```python
from build123d import *

# Parameters (mm, degrees)
SKETCH1_R                       = 48.5
SKETCH1_R_2                     = 1.5
BOSS_EXTRUDE3_DEPTH             = 4
BOSS_EXTRUDE4_START             = 4
SKETCH3_R                       = 9
BOSS_EXTRUDE4_DEPTH             = 14
CUT_EXTRUDE2_START              = 6
SKETCH5_R                       = 1.3
CUT_EXTRUDE2_DEPTH              = 96.333743786
BOSS_EXTRUDE5_DEPTH             = 9
BOSS_EXTRUDE5_DIRECTION_2_REACH = 113.079
CUT_EXTRUDE3_DEPTH              = 107.628687584
CUT_EXTRUDE3_DEPTH_BACK         = 107.628687584
FILLET1_R                       = 10
FILLET2_R                       = 2
SKETCH11_R                      = 3.75
CUT_EXTRUDE4_DEPTH              = 2.6


with BuildPart() as part:
    # Sketch1 → Boss-Extrude3 (new body)
    with BuildSketch(Plane(origin=(0, 0, 0), x_dir=(1, 0, 0), z_dir=(0, 1, 0))):
        with Locations(Location((0, 0, 0), (0, 0, 270))):
            Circle(SKETCH1_R)
        with Locations(Location((0, 7.25, 0), (0, 0, 270))):
            Circle(SKETCH1_R_2, mode=Mode.SUBTRACT)
        with Locations(Location((0, -7.25, 0), (0, 0, 270))):
            Circle(SKETCH1_R_2, mode=Mode.SUBTRACT)
    extrude(amount=BOSS_EXTRUDE3_DEPTH)

    # Sketch3 → Boss-Extrude4 (add)
    with BuildSketch(Plane(origin=(0, 0, 0), x_dir=(0, 0, -1), z_dir=(1, 0, 0)).offset(BOSS_EXTRUDE4_START)):
        with BuildLine():
            Line((30.34, 4), (-30.34, 4))
            Line((-30.34, 4), (-30.34, 11.86))
            ThreePointArc((-30.34, 11.86), (-29.573286886, 19.169908139), (-27.306519614, 26.161644128))
            Line((-27.306519614, 26.161644128), (-13.792358873, 56.58534489))
            ThreePointArc((-13.792358873, 56.58534489), (31.303559207, 69.105517077), (34.935565542, 22.444986978))
            ThreePointArc((34.935565542, 22.444986978), (31.536621485, 17.510838233), (30.34, 11.64))
            Line((30.34, 11.64), (30.34, 4))
        make_face()
        with Locations((13.91, 44.28)):
            Circle(SKETCH3_R, mode=Mode.SUBTRACT)
    extrude(amount=BOSS_EXTRUDE4_DEPTH)

    # Sketch5 → Cut-Extrude2 (cut, through all)
    with BuildSketch(Plane(origin=(0, 0, 0), x_dir=(0, 0, -1), z_dir=(1, 0, 0)).offset(CUT_EXTRUDE2_START)):
        with Locations(Location((27.167164466, 50.465339059, 0), (0, 0, 180))):
            Circle(SKETCH5_R)
        with Locations(Location((20.096096654, 57.536406871, 0), (0, 0, 180))):
            Circle(SKETCH5_R)
        with Locations(Location((-6.773961031, 16.524213562, 0), (0, 0, 180))):
            Circle(SKETCH5_R)
        with Locations(Location((-13.845028843, 23.595281374, 0), (0, 0, 180))):
            Circle(SKETCH5_R)
        Polygon((-0.41, 15.11), (28.581378029, 44.101378029), (13.732135624, 58.950620434), (-15.259242405, 29.959242405), align=None)
    extrude(amount=CUT_EXTRUDE2_DEPTH, mode=Mode.SUBTRACT)

    # Sketch9 → Boss-Extrude5 (add)
    with BuildSketch(Plane(origin=(18, 0, 0), x_dir=(0, 0, -1), z_dir=(1, 0, 0))):
        with BuildLine():
            Line((30.34, 4), (30.34, 11.64))
            ThreePointArc((30.34, 11.64), (31.536621485, 17.510838233), (34.935565542, 22.444986978))
            ThreePointArc((34.935565542, 22.444986978), (31.303559207, 69.105517077), (-13.792358873, 56.58534489))
            ThreePointArc((-13.792358873, 56.58534489), (-24.20389685, 31.229863028), (-27.34, 4))
            Line((-27.34, 4), (-36.34, 4))
            Line((-36.34, 4), (-36.34, 11.86))
            ThreePointArc((-36.34, 11.86), (-35.442708439, 20.414854175), (-32.789889403, 28.597348492))
            Line((-32.789889403, 28.597348492), (-19.275728663, 59.021049255))
            ThreePointArc((-19.275728663, 59.021049255), (34.746418262, 74.019448449), (39.097339325, 18.122992187))
            ThreePointArc((39.097339325, 18.122992187), (37.057972891, 15.16250294), (36.34, 11.64))
            Line((36.34, 11.64), (36.34, 4))
            Line((36.34, 4), (30.34, 4))
        make_face()
    extrude(amount=BOSS_EXTRUDE5_DEPTH)

    # Boss-Extrude5 direction 2: up to this face of the body (flat: up to its plane)
    boss_extrude5_direction_2_end = Plane(part.part.faces().sort_by_distance((4, 35.761181815, -7.797700276))[0])
    # Sketch9 → Boss-Extrude5 direction 2 (add, up to the picked face)
    with BuildSketch(Plane(origin=(18, 0, 0), x_dir=(0, 0, -1), z_dir=(1, 0, 0)), mode=Mode.PRIVATE) as boss_extrude5_direction_2_sk1:
        with BuildLine():
            Line((30.34, 4), (30.34, 11.64))
            ThreePointArc((30.34, 11.64), (31.536621485, 17.510838233), (34.935565542, 22.444986978))
            ThreePointArc((34.935565542, 22.444986978), (31.303559207, 69.105517077), (-13.792358873, 56.58534489))
            ThreePointArc((-13.792358873, 56.58534489), (-24.20389685, 31.229863028), (-27.34, 4))
            Line((-27.34, 4), (-36.34, 4))
            Line((-36.34, 4), (-36.34, 11.86))
            ThreePointArc((-36.34, 11.86), (-35.442708439, 20.414854175), (-32.789889403, 28.597348492))
            Line((-32.789889403, 28.597348492), (-19.275728663, 59.021049255))
            ThreePointArc((-19.275728663, 59.021049255), (34.746418262, 74.019448449), (39.097339325, 18.122992187))
            ThreePointArc((39.097339325, 18.122992187), (37.057972891, 15.16250294), (36.34, 11.64))
            Line((36.34, 11.64), (36.34, 4))
            Line((36.34, 4), (30.34, 4))
        make_face()
    boss_extrude5_direction_2_tool1 = split(extrude(boss_extrude5_direction_2_sk1.sketch, amount=-BOSS_EXTRUDE5_DIRECTION_2_REACH, mode=Mode.PRIVATE), bisect_by=boss_extrude5_direction_2_end, keep=Keep.BOTH, mode=Mode.PRIVATE)
    add(boss_extrude5_direction_2_tool1.solids().sort_by(Axis((18, 43.339989, 24.976501), (-1, 0, 0)))[0])

    # Sketch10 → Cut-Extrude3 (cut, two sides: drawn at the far end of the back side and taken through both)
    with BuildSketch(Plane.XY.offset(-CUT_EXTRUDE3_DEPTH_BACK)):
        with BuildLine():
            Line((27, 80.59241), (21, 80.59241))
            ThreePointArc((21, 80.59241), (22.277450308, 42.190463148), (26.5, 4))
            Line((26.5, 4), (27, 4))
            Line((27, 4), (27, 80.59241))
        make_face()
    extrude(amount=CUT_EXTRUDE3_DEPTH + CUT_EXTRUDE3_DEPTH_BACK, mode=Mode.SUBTRACT)

    # Fillet1
    # the kernel refuses this fillet: 10 mm, written as the material it takes off along each edge
    with BuildSketch(Plane(origin=(4, 11.64, -36.34), x_dir=(0, 0, 1), z_dir=(0, -1, 0))) as fillet1_piece_1:
        with BuildLine():
            CenterArc((FILLET1_R, -FILLET1_R), FILLET1_R, 90, 90)
            Line((0, -FILLET1_R), (0, 0))
            Line((0, 0), (FILLET1_R, 0))
        make_face()
    extrude(amount=7.64, mode=Mode.SUBTRACT)
    with BuildSketch(Plane(origin=(4, 11.64, -45.34), x_dir=(0, 0.7203324652134895, 0.6936289638988969), z_dir=(0, 0.6936289638988969, -0.7203324652134895))) as fillet1_piece_2:
        with BuildLine():
            CenterArc((9 + FILLET1_R, FILLET1_R), FILLET1_R, 180, 90)
            Line((9, FILLET1_R), (9, 0))
            Line((9, 0), (9 + FILLET1_R, 0))
        make_face()
    revolve(axis=Axis((4, 11.64, -45.34), (1, 0, 0)), revolution_arc=46.081936205, mode=Mode.SUBTRACT)
    with BuildSketch(Plane(origin=(4, 44.28, -13.91), x_dir=(0, -0.7203324652134897, -0.6936289638988965), z_dir=(0, -0.6936289638988965, 0.7203324652134897))) as fillet1_piece_3:
        with BuildLine():
            CenterArc((36.31241 - FILLET1_R, FILLET1_R), FILLET1_R, 270, 90)
            Line((36.31241, FILLET1_R), (36.31241, 0))
            Line((36.31241, 0), (36.31241 - FILLET1_R, 0))
        make_face()
    revolve(axis=Axis((4, 44.28, -13.91), (1, 0, 0)), revolution_arc=202.131217863, mode=Mode.SUBTRACT)
    with BuildSketch(Plane(origin=(4, 28.597348492, 32.789889403), x_dir=(0, -0.40595072743967076, -0.913894964911834), z_dir=(0, 0.913894964911834, -0.4059507274396708))) as fillet1_piece_4:
        with BuildLine():
            CenterArc((FILLET1_R, -FILLET1_R), FILLET1_R, 90, 90)
            Line((0, -FILLET1_R), (0, 0))
            Line((0, 0), (FILLET1_R, 0))
        make_face()
    extrude(amount=33.290150324, mode=Mode.SUBTRACT)
    with BuildSketch(Plane(origin=(4, 11.86, -4.89), x_dir=(0, 0.4059507274396698, 0.9138949649118343), z_dir=(0, 0.9138949649118343, -0.4059507274396698))) as fillet1_piece_5:
        with BuildLine():
            CenterArc((41.23 - FILLET1_R, FILLET1_R), FILLET1_R, 270, 90)
            Line((41.23, FILLET1_R), (41.23, 0))
            Line((41.23, 0), (41.23 - FILLET1_R, 0))
        make_face()
    revolve(axis=Axis((4, 11.86, -4.89), (1, 0, 0)), revolution_arc=23.950718343, mode=Mode.SUBTRACT)
    with BuildSketch(Plane(origin=(4, 4, 36.34), x_dir=(0, 0, -1), z_dir=(0, 1, 0))) as fillet1_piece_6:
        with BuildLine():
            CenterArc((FILLET1_R, -FILLET1_R), FILLET1_R, 90, 90)
            Line((0, -FILLET1_R), (0, 0))
            Line((0, 0), (FILLET1_R, 0))
        make_face()
    extrude(amount=7.86, mode=Mode.SUBTRACT)

    # Fillet2
    fillet2_edges = [part.edges().sort_by_distance(p)[0] for p in [
        (20.25, 4, -36.34),
        (20.25, 4, 36.34),
        (6.928932188, 4, 33.411067812),
        (4, 4, 0),
        (6.928932188, 4, -33.411067812),
    ]]
    fillet(fillet2_edges, radius=FILLET2_R)
    fillet2_2_edges = [part.edges().sort_by_distance(p)[0] for p in [
        (26.5, 4, -33.34),
    ]]
    fillet(fillet2_2_edges, radius=FILLET2_R)
    fillet2_3_edges = [part.edges().sort_by_distance(p)[0] for p in [
        (26.5, 4, 31.84),
    ]]
    fillet(fillet2_3_edges, radius=FILLET2_R)

    # Sketch11 → Cut-Extrude4 (cut)
    with BuildSketch(Plane.XZ):
        with Locations(Location((0, 0, 0), (0, 0, 270))):
            Circle(SKETCH11_R)
    extrude(amount=-CUT_EXTRUDE4_DEPTH, mode=Mode.SUBTRACT)


solid = part.part
```
For this review, take the finished solid that the model builds, in its own axes (mm). A direction names the side the tool comes from. Round coordinates to 2 decimals unless told otherwise and drop trailing zeros. Write each loop counter-clockwise with the first axis right and the second up, starting at its lowest first coordinate (ties: lowest second). Pieces come first, ordered by that corner, then holes.
1) Mouldability with a two-part tool opening along Z and no side actions: class faces 5 (the face through (6.852, 42.375, 23.379)), 6 (the face through (20, 9, -36.34)), 7 (the face through (6, 50, -27)) as +Z half, -Z half, draft (parallel to the pull), parting line (faces both ways), or undercut.
Answer below:
face 5: +Z half
face 6: -Z half
face 7: undercut
2) Take a section at A-A on x = 0. Give the boundary of the cut face in (y, z), then the cut area to 4 significant figures.
Answer below:
outline: (0, -48.5) - (4, -48.5) - (4, -8.75) - (0, -8.75) - close; (0, -5.75) - (4, -5.75) - (4, 5.75) - (0, 5.75) - (0, 3.75) - (2.6, 3.75) - (2.6, -3.75) - (0, -3.75) - close; (0, 8.75) - (4, 8.75) - (4, 48.5) - (0, 48.5) - close
area: 344.5 mm2
3) Insertion check: pin 1 Ø1.8 at (x, y) = (18, 9) entering from +Z; pin 2 Ø6 at (x, y) = (4.5, 46) entering from +Z; pin 3 Ø2.5 at (y, z) = (23.6, 13.85) entering from +X; pin 4 Ø2.5 at (x, z) = (0, 7.25) entering from +Y. Each pin has a flat end and moves straight along its axis. Give the tip position at first contact, or say it passes through.
Answer below:
pin 1: stops at z = 36.34
pin 2: stops at z = 22.72
pin 3: stops at x = 6
pin 4: passes through
4) For line 1 along X through (y, z) = (52.5, -38.5); line 2 along Y through (x, z) = (-0.5, -13.5); line 3 along Y through (x, z) = (17, -17), list the stretches that pass through material, from the lowest coordinate up.
Answer below:
line 1: x = 4 to 18
line 2: y = 0 to 4
line 3: y = 0 to 32.52, 55.68 to 80.46
5) Machinability: for faces 1 (the face through (6.85, 8.89, 33.33)), 2 (the face through (6.85, 8.86, -33.33)), 3 (the face through (11.92, 29.4, -13.88)), 4 (the face through (0, 2.6, 0)), which of the approach directions +Z, -Z, +X, -X, +Y, -Y give a long, thin tool a straight path to every point of the face, cutting with its end or side? Answer none if there is none.
Answer below:
face 1: +Z, -X, +Y
face 2: -Z, -X
face 3: +X
face 4: -Y
6) Take a section at B-B on z = -7.25. State how many separate pieces and enclosed holes the cut face has, then the cut area to 3 significant figures.
Answer below:
separate pieces: 3
enclosed holes: 0
area: 1,050 mm2
